Design review of the part built by this model. Coordinates are the model's own, in mm. A direction names the side the tool comes from. Coordinates: 2 decimals unless noted, no trailing zeros. Order: outer loops, then holes, each group sorted by start corner. A loop starts at its lowest first (then second) coordinate and runs counter-clockwise, first axis right, second up. Notation, with made-up numbers: (79.5, 61.25) - (114.5, 61.25) arc R8 ccw to (114.5, 71.25) - close; hole circle Ø10 at (-32.75, 86.25). An arc over 180 degrees is marked (long way). Write each question's results on one line, items separated by ' | '. Start each with the question number.
```python
from build123d import *

# Parameters (mm, degrees)
F1_DEPTH = 115


with BuildPart() as f1:
    # F0 (on Right) → F1 (new body)
    with BuildSketch(Plane.YZ):
        with BuildLine():
            Line((-89.63947, 6.738275), (-114.754856, 0))
            Line((-114.754856, 0), (-138.194978, -5.876377))
            Line((-138.194978, -5.876377), (-156.873196, -15.215486))
            Line((-156.873196, -15.215486), (-149.503788, -29.954302))
            Line((-149.503788, -29.954302), (-123.761818, -39.761275))
            Line((-123.761818, -39.761275), (-108.140029, -39.761275))
            ThreePointArc((-108.140029, -39.761275), (-102.198985, -25.605666), (-88.001989, -19.764215))
            ThreePointArc((-88.001989, -19.764215), (-73.834486, -25.845282), (-67.198023, -39.761275))
            Line((-67.198023, -39.761275), (-37.212595, -39.761275))
            Line((-37.212595, -39.761275), (72.381705, -39.761275))
            ThreePointArc((72.381705, -39.761275), (78.034801, -25.038001), (92.89816, -19.764215))
            ThreePointArc((92.89816, -19.764215), (106.193601, -26.50791), (111.596704, -40.402249))
            Line((111.596704, -40.402249), (127.211124, -40.402249))
            Line((127.211124, -40.402249), (146.114811, -31.879209))
            Line((146.114811, -31.879209), (146.114811, -15.81654))
            Line((146.114811, -15.81654), (140.074372, -15.81654))
            Line((140.074372, -15.81654), (140.074372, 4.835445))
            Line((140.074372, 4.835445), (147.833586, 12.251377))
            Line((147.833586, 12.251377), (140.074372, 12.251377))
            Line((140.074372, 12.251377), (108.220726, 12.251377))
            Line((108.220726, 12.251377), (94.54, 18.989645))
            Line((94.54, 18.989645), (74.325174, 30.015916))
            Line((74.325174, 30.015916), (49.209803, 37.162594))
            Line((49.209803, 37.162594), (22.869274, 36.754213))
            Line((22.869274, 36.754213), (-7.963434, 32.466225))
            Line((-7.963434, 32.466225), (-30.220151, 21.235771))
            Line((-30.220151, 21.235771), (-55.131346, 6.738275))
            Line((-55.131346, 6.738275), (-89.63947, 6.738275))
        make_face()
    extrude(amount=F1_DEPTH)


solid = f1.part
```
(1) Mouldability with a two-part tool opening along Z and no side actions: class faces 1 (the face through (56.7, 84.57, 24.43)), 2 (the face through (57, 140.074, -6)), 3 (the face through (56.7, -102.35, -25.76)) as +Z half, -Z half, draft (parallel to the pull), parting line (faces both ways), or undercut.
(2) Tool access review of faces 4 (the face through (56.7, 143.9, 8.49)), 5 (the face through (57, 128, 12.251)), 6 (the face through (56.695, -73.994, -25.693)), 7 (the face through (57, 146.115, -24)): name each direction out of +Z, -Z, +X, -X, +Y, -Y from which nothing blocks a thin tool from reaching the whole face with its end or side.
(3) To check wall thickness, follow line 1 along Y through (x, z) = (87, -29); line 2 along Y through (x, z) = (10.5, -22); line 3 along Z through (x, y) = (25, -56.5). State the ranges of each line that lie inside material, in increasing order. Write a range as [from, to].
(4) Take a section at D-D (z = 15). State the section outline as (x, y) points, plus the area to 3 significant figures.
(5) Take a section at C-C (y = -4). State the section outline as (x, z) points.
(6) Take a section at B-B (x = 75.5). State the section outline as (y, z) points, plus the area to 3 significant figures.
(7) Clearance check with flat-ended pins moving along their axes: pin 1 (12.5 mm diameter, centred on x = 74.5, y = -113, fed in from -Z); pin 2 (1 mm diameter, centred on y = 69, z = -10.5, fed in from -X); pin 3 (17.5 mm diameter, centred on x = 40.5, y = -65, fed in from +Z); pin 4 (10 mm diameter, centred on x = 89.5, z = 6, fed in from +Y). State where each tip first meets the part, or that it passes through.
(8) Take a section at A-A (z = -26). State the section outline as (x, y) points, plus the area to 3 significant figures.
Worked out:
1) face 1: +Z half | face 2: undercut | face 3: -Z half
2) face 4: +X, -X, +Y | face 5: +Z, +X, -X, +Y | face 6: -Z, +X, -X | face 7: -Z, +X, -X, +Y
3) line 1: [-149.98, -104.94], [-71.12, 74.93], [108.13, 146.11] | line 2: [-153.48, -97.24], [-79.31, 82.14], [100.35, 146.11] | line 3: [-39.76, 6.74]
4) outline: (0, -40.94) - (115, -40.94) - (115, 102.64) - (0, 102.64) - close | area: 16,500 mm^2
5) outline: (0, -39.76) - (115, -39.76) - (115, 33.02) - (0, 33.02) - close
6) outline: (-156.87, -15.22) - (-149.5, -29.95) - (-123.76, -39.76) - (-108.14, -39.76) arc R20.11 cw to (-88, -19.76) arc R21.87 cw to (-67.2, -39.76) - (72.38, -39.76) arc R18.85 cw to (92.9, -19.76) arc R20.87 cw to (111.6, -40.4) - (127.21, -40.4) - (146.11, -31.88) - (146.11, -15.82) - (140.07, -15.82) - (140.07, 4.84) - (147.83, 12.25) - (108.22, 12.25) - (94.54, 18.99) - (74.33, 30.02) - (49.21, 37.16) - (22.87, 36.75) - (-7.96, 32.47) - (-30.22, 21.24) - (-55.13, 6.74) - (-89.64, 6.74) - (-114.75, 0) - (-138.19, -5.88) - close | area: 15,400 mm^2
7) pin 1: z = -39.76 | pin 2: x = 0 | pin 3: z = 6.74 | pin 4: y = 146.52
8) outline: (0, -151.48) - (115, -151.48) - (115, -102.59) - (0, -102.59) - close; (0, -73.68) - (115, -73.68) - (115, 77.12) - (0, 77.12) - close; (0, 105.72) - (115, 105.72) - (115, 146.11) - (0, 146.11) - close | area: 27,600 mm^2
